Verification items for this drawing (mm, ordinates from the low corner). Round coordinates to 2 decimals unless told otherwise and drop trailing zeros. Loops run counter-clockwise (first coordinate to the right, second up) from the corner with the lowest first, then second, coordinate; pieces in that order, holes last. Notation, with made-up numbers: M 78,-20 L 94,-20 A21 cw 94,-4 Z; hole C 71,76 d7. An arc over 180 degrees is marked long. Write item = value, one per line. Start each with the question number.
(1) Go/stop test with a flat-tipped pin: P1, Ø1, axis at x = 64, z = 2, coming from the +Y side. Record where the tip stops, or that it passes through.
(2) Cross-section at A-A on x = 46.2. Record the boundary of the cut face in (y, z).
(3) Cross-section at D-D on z = 0.35. Record the boundary of the cut face in (x, y) (1 decimal).
(4) Scan lines: L1, parallel to X at y = 58, z = 0.4 (1 decimal); L2, parallel to Y at x = 57.5, z = 0.5 (1 decimal); L3, parallel to X at y = 76.5, z = 0.8 (1 decimal). Record each from-to range of solid material in increasing order. Write a range as from..to.
(5) Cross-section at C-C on x = 57. Record the boundary of the cut face in (y, z).
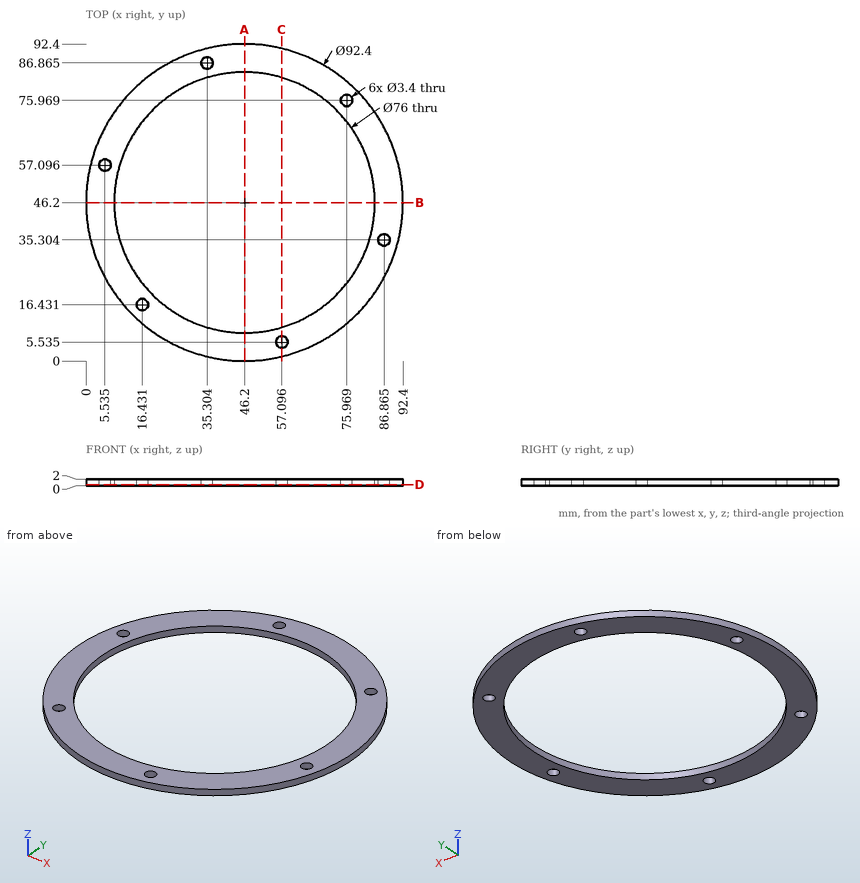
Result:
q1.P1 = 89.04
q2.outline = M 0,0 L 8.2,0 L 8.2,2 L 0,2 Z; M 84.2,0 L 92.4,0 L 92.4,2 L 84.2,2 Z
q3.outline = C 46.2,46.2 d92.4; hole C 5.5,57.1 d3.4; hole C 46.2,46.2 d76; hole C 16.4,16.4 d3.4; hole C 35.3,86.9 d3.4; hole C 57.1,5.5 d3.4; hole C 76,76 d3.4; hole C 86.9,35.3 d3.4
q4.L1 = 1.5..4.1, 7..10.1, 82.3..90.9
q4.L2 = 1.4..3.9, 7.2..9.9, 82.5..91
q4.L3 = 11.3..23.3, 69.1..74.4, 77.6..81.1
q5.outline = M 1.28,0 L 3.84,0 L 3.84,2 L 1.28,2 Z; M 7.23,0 L 9.77,0 L 9.77,2 L 7.23,2 Z; M 82.63,0 L 91.12,0 L 91.12,2 L 82.63,2 Z
